Geometry: see drawing. Coordinates: mm, zero at the bounding-box minimum. Give positions to 0.01 mm unless a question says otherwise; leave off trailing zeros. Loops run counter-clockwise (first coordinate to the right, second up) from the corner with the lowest first, then second, coordinate; pieces in that order, holes last. Notation, with made-up numbers: (75.5, -2.75) - (100.5, -2.75) arc R5 cw to (100.5, 3.25) - close; hole circle Ø10 at (-35, -31). An arc over 180 degrees is marked (long way). Use one line per item in the form item = value.
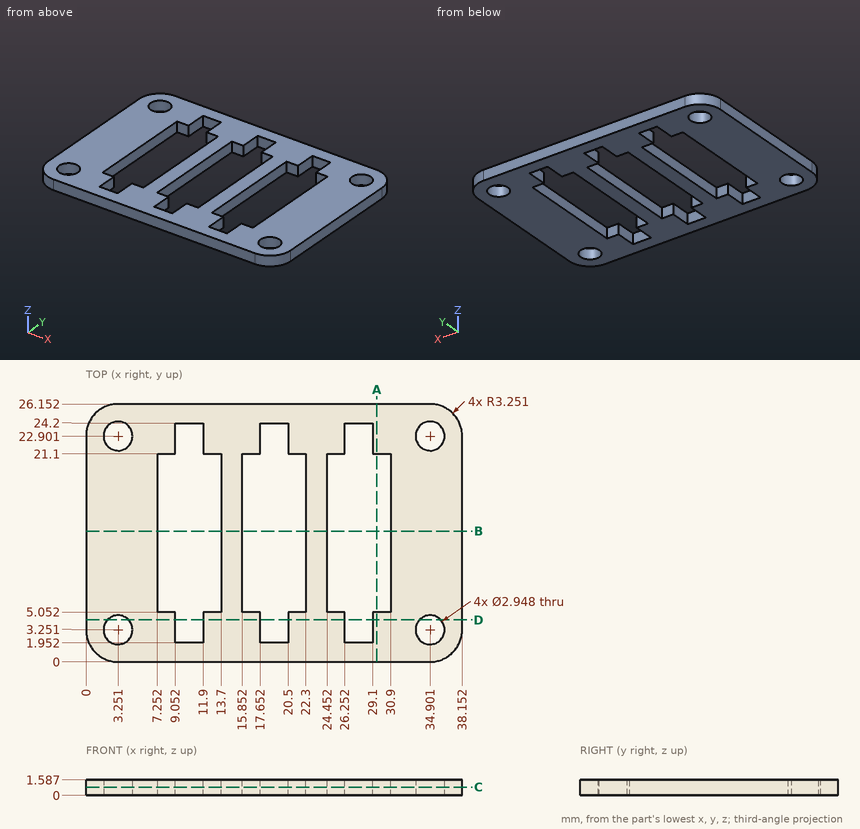
(1) Material intervals for L1, parallel to X at y = 15.5, z = 0.1; L2, parallel to X at y = 23, z = 0.5; L3, parallel to Y at x = 19.5, z = 1.4, sorted ascending. Write a range as from..to.
Solution:
L1 = 0..7.25, 13.7..15.85, 22.3..24.45, 30.9..38.15
L2 = 0..1.78, 4.72..9.05, 11.9..17.65, 20.5..26.25, 29.1..33.43, 36.37..38.15
L3 = 0..1.95, 24.2..26.15
(2) Pin query (flat end, axial travel): P1, Ø2.5, axis at x = 34.9, y = 22.9, coming from the +Z side. Return the tip coordinate at first contact, or that it passes through.
Solution:
P1 = through
(3) Cut plane A-A (x = 29.5). Return the cut outline in (y, z).
Solution:
outline = (0, 0) - (5.05, 0) - (5.05, 1.59) - (0, 1.59) - close; (21.1, 0) - (26.15, 0) - (26.15, 1.59) - (21.1, 1.59) - close
(4) Cut plane D-D (y = 4.25). Return the cut outline in (x, z) (1 decimal).
Solution:
outline = (0, 0) - (2.2, 0) - (2.2, 1.6) - (0, 1.6) - close; (4.3, 0) - (9.1, 0) - (9.1, 1.6) - (4.3, 1.6) - close; (11.9, 0) - (17.7, 0) - (17.7, 1.6) - (11.9, 1.6) - close; (20.5, 0) - (26.3, 0) - (26.3, 1.6) - (20.5, 1.6) - close; (29.1, 0) - (33.8, 0) - (33.8, 1.6) - (29.1, 1.6) - close; (36, 0) - (38.2, 0) - (38.2, 1.6) - (36, 1.6) - close
(5) Cut plane C-C (z = 0.85). Give the number of separate pieces and of enclosed holes in the cut face, plus the area to 3 significant figures.
Solution:
separate_pieces = 1
enclosed_holes = 7
area = 598 mm2
(6) Cut plane B-B (y = 13.25). Return the cut outline in (x, z).
Solution:
outline = (0, 0) - (7.25, 0) - (7.25, 1.59) - (0, 1.59) - close; (13.7, 0) - (15.85, 0) - (15.85, 1.59) - (13.7, 1.59) - close; (22.3, 0) - (24.45, 0) - (24.45, 1.59) - (22.3, 1.59) - close; (30.9, 0) - (38.15, 0) - (38.15, 1.59) - (30.9, 1.59) - close
